Part model, mm, in its own coordinate system. Give positions to 0.01 mm unless a question says otherwise; leave off trailing zeros. Write each loop counter-clockwise with the first axis right and the second up, starting at its lowest first coordinate (ties: lowest second). Pieces come first, ordered by that corner, then holes.
Autodesk Inventor part; units mm, degrees
ref_plane "YZ Plane" through (0, 0, 0) normal (1, 0, 0) x (0, 1, 0)
ref_plane "XZ Plane" through (0, 0, 0) normal (0, 1, 0) x (-1, 0, 0)
ref_plane "XY Plane" through (0, 0, 0) normal (0, 0, 1) x (1, 0, 0)
sketch "Sketch1" plane through (0, 0, 0) normal (0, 0, 1) x (1, 0, 0)
  line L0 (-36.5125, 12.7) -> (36.5125, 12.7)
  line L1 (36.5125, 12.7) -> (36.5125, -12.7)
  line L2 (36.5125, -12.7) -> (-36.5125, -12.7)
  line L3 (-36.5125, -12.7) -> (-36.5125, 12.7)
  line L4 (-36.5125, 12.7) -> (36.5125, -12.7) construction
  line L5 (36.5125, 12.7) -> (-36.5125, -12.7) construction
  point P0 (0, 0)
  dimension "d15" = 73.025
  dimension "d16" = 25.4
extrude "Extrusion1" add sketch "Sketch1" along normal blind 3.175
sketch "Sketch3" plane through (0, 0, 3.175) normal (0, 0, 1) x (1, 0, 0)
  line L0 (-36.5125, 12.7) -> (-36.5125, -12.7)
  line L1 (36.5125, -12.7) -> (36.5125, 12.7)
  point P0 (0, 0)
  point P1 (23.8125, 0)
  point P2 (-1.7145, 0)
  point P3 (36.5125, 0)
  dimension "d17" = 25.527
  dimension "d27" = 12.7
hole "Hole2" at (23.8125, 0, 3.175) at (-1.7145, 0, 3.175) direction (0, 0, -1) diameter 5.1054 end through all
fillet "Fillet2" radius 3.175 4 edges at (-36.5125, 12.7, 1.5875) (-36.5125, -12.7, 1.5875) (36.5125, 12.7, 1.5875) (36.5125, -12.7, 1.5875)
properties part number "EL2-016" material "Aluminum 6061"
1) Saw through at A-A (y = 0). Write the cut outline in (x, z) (1 decimal), and give its area (3 significant figures).
Check result:
outline: (-36.5, 0) - (-4.3, 0) - (-4.3, 3.2) - (-36.5, 3.2) - close; (0.8, 0) - (21.3, 0) - (21.3, 3.2) - (0.8, 3.2) - close; (26.4, 0) - (36.5, 0) - (36.5, 3.2) - (26.4, 3.2) - close
area: 199 mm2
2) Drill centre lines: L1, parallel to X at y = 0, z = 1; L2, parallel to X at y = -2, z = 1.25; L3, parallel to Y at x = 24, z = 1.1. Where is each one in solid material? Low to high.
Check result:
L1: x = -36.51 to -4.27, 0.84 to 21.26, 26.37 to 36.51
L2: x = -36.51 to -3.3, -0.13 to 22.23, 25.4 to 36.51
L3: y = -12.7 to -2.55, 2.55 to 12.7
3) Saw through at B-B (x = -3.5). Write the cut outline in (y, z) (3 decimals), and give its area (3 significant figures).
Check result:
outline: (-12.7, 0) - (-1.824, 0) - (-1.824, 3.175) - (-12.7, 3.175) - close; (1.824, 0) - (12.7, 0) - (12.7, 3.175) - (1.824, 3.175) - close
area: 69.1 mm2
4) Saw through at C-C (z = 0.5). State how many separate pieces and enclosed holes the cut face has, and give its area (3 significant figures).
Check result:
separate pieces: 1
enclosed holes: 2
area: 1,810 mm2
5) Mould opens along Y. For faces 1 (the flat face through (36.512, 0, 2)), 2 (the cylindrical face through (21.66, -1.37, 1.57)), 3 (the cylindrical face through (-2.481, -2.435, 1.565)), 4 (the flat face through (0, -12.7, 2)) say: +Y half, -Y half, draft (parallel to the pull), parting line (faces both ways), or undercut.
Check result:
face 1: draft
face 2: undercut
face 3: undercut
face 4: -Y half
